Drawing for the job (mm, zero at the part's lowest x, y, z). Round coordinates to 2 decimals unless told otherwise and drop trailing zeros. Loops run counter-clockwise (first coordinate to the right, second up) from the corner with the lowest first, then second, coordinate; pieces in that order, holes last. Notation, with made-up numbers: M 55.25,32.25 L 62.25,32.25 A31 cw 62.25,70.25 Z; hole C 86,-37.75 d9. An arc over 180 degrees is marked long. Write each question's results on one line, items separated by ' | '.
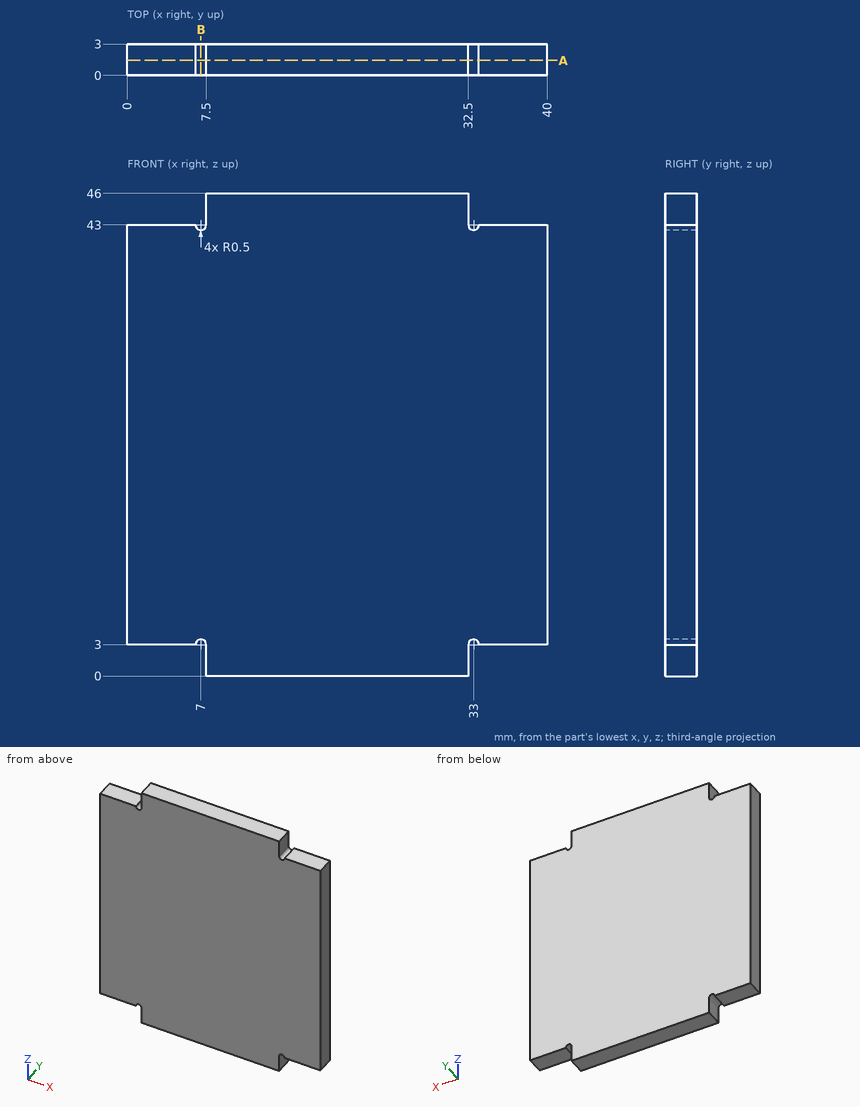
Item 1: Band-saw the part on A-A on y = 1.45. Give the cut face in (x, z).
Filled sheet:
outline: M 0,3 L 6.5,3 A0.5 cw 7.5,3 L 7.5,0 L 32.5,0 L 32.5,3 A0.5 cw 33.5,3 L 40,3 L 40,43 L 33.5,43 A0.5 cw 32.5,43 L 32.5,46 L 7.5,46 L 7.5,43 A0.5 cw 6.5,43 L 0,43 Z
Item 2: Wall check: L1, parallel to Z at x = 3, y = 0.2. Give the ranges that are in metal, low to high.
Filled sheet:
L1: 3 to 43
Item 3: Band-saw the part on B-B on x = 7. Give the cut face in (y, z).
Filled sheet:
outline: M 0,3.5 L 3,3.5 L 3,42.5 L 0,42.5 Z
Item 4: Drop flat-ended pins along their axis: P1, Ø0.9, axis at y = 2, z = 1.5, coming from the -X side; P2, Ø0.9, axis at y = 1, z = 45, coming from the +X side; P3, Ø0.9, axis at x = 36.5, y = 2, coming from the +Z side. Give the stop position or say it passes through.
Filled sheet:
P1: x = 7.5 | P2: x = 32.5 | P3: z = 43
